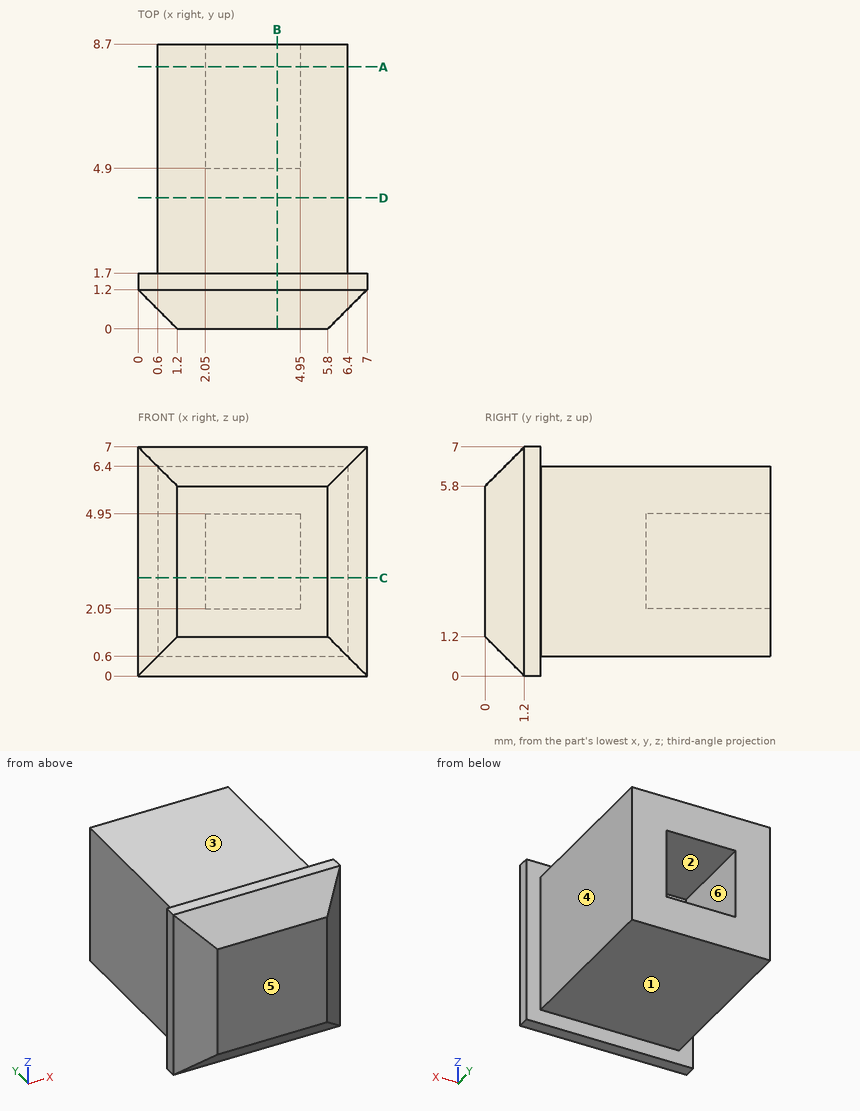
For this review, use the dimensioned drawing (mm, ordinates from the lowest corner) and the shaded views. A direction names the side the tool comes from. Round coordinates to 2 decimals unless told otherwise and drop trailing zeros. Order: outer loops, then holes, each group sorted by start corner. A loop starts at its lowest first (then second) coordinate and runs counter-clockwise, first axis right, second up. Notation, with made-up numbers: (82, 64) -> (105, 64) arc R16 ccw to (105, 73) -> close; hole circle Ø2 at (-33.75, 84). An arc over 180 degrees is marked (long way). Use CSV: the item, a comma, the result in double quotes. Start each with the question number.
(1) Wall thickness on probe 1 along Z at (x, y) = (4.5, 6); probe 2 along X at (y, z) = (8.25, 0.75): over which ranges is each line inside the solid? List them lowest first. Write a range as from..to.
(2) Insertion check: pin 1 (0.9 mm diameter, centred on x = 3, y = 6.5, fed in from -Z); pin 2 (1.5 mm diameter, centred on x = 3, z = 3.5, fed in from +Y); pin 3 (2 mm diameter, centred on y = 2.5, z = 6.5, fed in from +X); pin 4 (1.7 mm diameter, centred on y = 5.5, z = 4.5, fed in from +X). Each pin has a flat end and moves straight along its axis. Give the tip position at first contact, or say it passes through.
(3) Consider section A-A on y = 8. Write out the cut boundary in (x, z), and give its area (3 significant figures).
(4) Tool access review of the marked faces 1, 2 and 3: name each direction out of +Z, -Z, +X, -X, +Y, -Y from which nothing blocks a thin tool from reaching the whole face with its end or side.
(5) Mouldability with a two-part tool opening along X and no side actions: class the marked faces 4, 5 and 6 as pulls with the +X half, pulls with the -X half, needs draft (parallel to the pull), parting line crosses it, or undercut.
(6) Consider section B-B on x = 4.25. Write out the cut boundary in (y, z), and give its area (3 significant figures).
(7) Consider section C-C on z = 3. Write out the cut boundary in (x, y), and give its area (3 significant figures).
(8) Consider section D-D on y = 4. Write out the cut boundary in (x, z), and give its area (3 significant figures).
Responses:
1,probe 1,"0.6..2.05, 4.95..6.4"
1,probe 2,"0.6..6.4"
2,pin 1,"z = 0.6"
2,pin 2,"y = 4.9"
2,pin 3,"x = 7"
2,pin 4,"x = 6.4"
3,outline,"(0.6, 0.6) -> (6.4, 0.6) -> (6.4, 6.4) -> (0.6, 6.4) -> close; hole (2.05, 2.05) -> (4.95, 2.05) -> (4.95, 4.95) -> (2.05, 4.95) -> close"
3,area,"25.2 mm²"
4,face 1,"-Z, +X, -X, +Y"
4,face 2,"+Y"
4,face 3,"+Z, +X, -X, +Y"
5,face 4,"pulls with the +X half"
5,face 5,"needs draft"
5,face 6,"undercut"
6,outline,"(0, 1.2) -> (1.2, 0) -> (1.7, 0) -> (1.7, 0.6) -> (8.7, 0.6) -> (8.7, 2.05) -> (4.9, 2.05) -> (4.9, 4.95) -> (8.7, 4.95) -> (8.7, 6.4) -> (1.7, 6.4) -> (1.7, 7) -> (1.2, 7) -> (0, 5.8) -> close"
6,area,"40.0 mm²"
7,outline,"(0, 1.2) -> (1.2, 0) -> (5.8, 0) -> (7, 1.2) -> (7, 1.7) -> (6.4, 1.7) -> (6.4, 8.7) -> (4.95, 8.7) -> (4.95, 4.9) -> (2.05, 4.9) -> (2.05, 8.7) -> (0.6, 8.7) -> (0.6, 1.7) -> (0, 1.7) -> close"
7,area,"40.0 mm²"
8,outline,"(0.6, 0.6) -> (6.4, 0.6) -> (6.4, 6.4) -> (0.6, 6.4) -> close"
8,area,"33.6 mm²"
